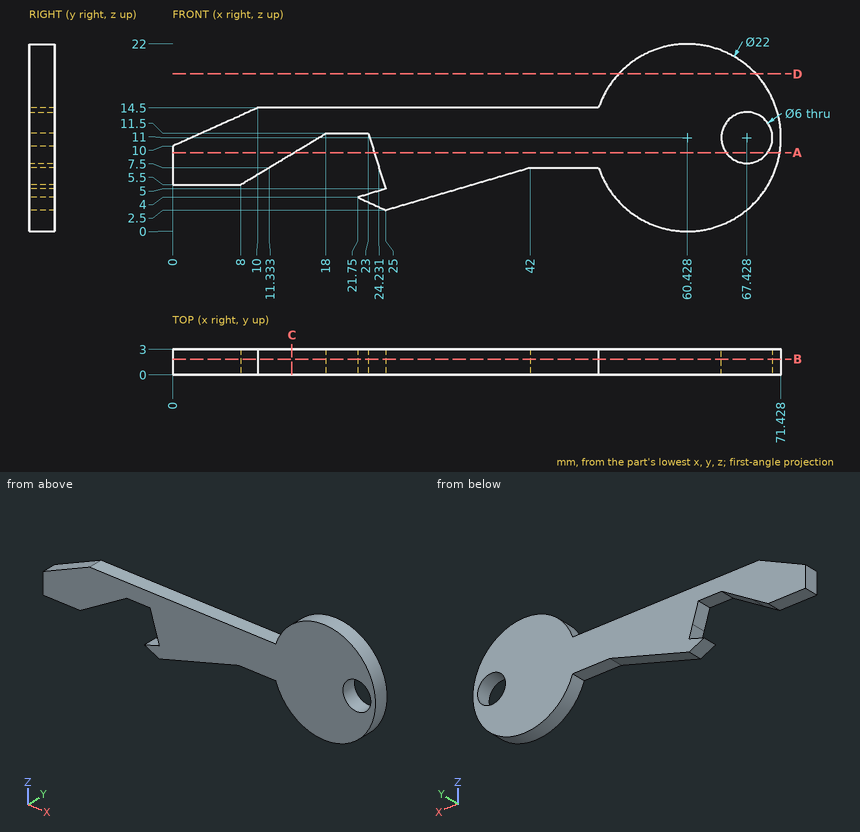
Here's the drawing with two shaded views (mm, measured from the low corner). I have some questions. Give positions to 0.01 mm unless a question says otherwise; leave off trailing zeros. Write each loop counter-clockwise with the first axis right and the second up, starting at its lowest first coordinate (ties: lowest second). Pieces come first, ordered by that corner, then holes. Notation, with made-up numbers: (-26.5, 82.25) -> (-9.5, 82.25) arc R27 ccw to (-9.5, 113.25) -> close; hole circle Ø10 at (30, -20.5). An arc over 180 degrees is marked (long way). Answer as a JSON object with one key per item and string values. Group by question number.
Item 1: Please list where these lines run through material, in increasing order: line 1 (X direction, y = 2.2, z = 11) (1 decimal); line 2 (Z direction, x = 60, y = 2); line 3 (Z direction, x = 66, y = 0.55) (1 decimal). Write a range as [from, to].
Item 2: I'm going to push flat-ended pins straight in: P1, Ø0.9, axis at x = 5.5, y = 1, coming from the -Z side; P2, Ø0.9, axis at x = 44.5, y = 1.5, coming from the -Z side. Where does each tip first touch, or does it pass through?
Item 3: Suppose I cut it at C-C (x = 14). Please give me the cut outline in (y, z), plus the area to 3 significant figures.
Item 4: Suppose I cut it at A-A (z = 9.25). State how many separate pieces and enclosed holes the cut face has, plus the area to 3 significant figures.
Item 5: Suppose I cut it at D-D (z = 18.5). Please give me the cut outline in (x, y) (1 decimal).
Item 6: Suppose I cut it at B-B (y = 1.85). Please give me the cut outline in (x, z).
Findings:
{
 "1": {"line 1": "x = [2.2, 17.2], [23.2, 64.4], [70.4, 71.4]", "line 2": "z = [0.01, 21.99]", "line 3": "z = [1.5, 8.4], [13.6, 20.5]"},
 "2": {"P1": "stops at z = 5.5", "P2": "stops at z = 7.5"},
 "3": {"outline": "(0, 9.1) -> (3, 9.1) -> (3, 14.5) -> (0, 14.5) -> close", "area": "16.2 mm²"},
 "4": {"separate pieces": "3", "enclosed holes": "0", "area": "171 mm²"},
 "5": {"outline": "(52.4, 0) -> (68.5, 0) -> (68.5, 3) -> (52.4, 3) -> close"},
 "6": {"outline": "(0, 5.5) -> (8, 5.5) -> (18, 11.5) -> (23, 11.5) -> (25, 5) -> (21.75, 4) -> (25, 2.5) -> (42, 7.5) -> (50, 7.5) arc R11 ccw (long way) to (50, 14.5) -> (10, 14.5) -> (0, 10) -> close; hole circle Ø6 at (67.43, 11)"}
}
